from build123d import *

# Parameters (mm, degrees)
SKETCH1_W           = 127
SKETCH1_H           = 52.832
BOSS_EXTRUDE1_DEPTH = 4.7625
FILLET1_R           = 2.54
SKETCH2_R           = 2.69
CUT_EXTRUDE1_DEPTH  = 69.940093286
SKETCH3_R           = 8.250000011
CUT_EXTRUDE2_DEPTH  = 69.940093286
SKETCH4_R           = 8.255000001
SKETCH4_R_2         = 3.450513254
CUT_EXTRUDE3_DEPTH  = 69.940093286


with BuildPart() as part:
    # Sketch1 → Boss-Extrude1 (new body)
    with BuildSketch(Plane(origin=(0, 0, 0), x_dir=(1, 0, 0), z_dir=(0, 1, 0))):
        Rectangle(SKETCH1_W, SKETCH1_H)
    extrude(amount=BOSS_EXTRUDE1_DEPTH)

    # Fillet1
    fillet1_edges = [part.edges().sort_by_distance(p)[0] for p in [
        (63.5, 2.38125, 26.416),
        (-63.5, 2.38125, 26.416),
        (-63.5, 2.38125, -26.416),
        (63.5, 2.38125, -26.416),
    ]]
    fillet(fillet1_edges, radius=FILLET1_R)

    # Sketch2 → Cut-Extrude1 (cut, through all)
    with BuildSketch(Plane.XZ):
        with Locations(Location((57.15, -15.24, 0), (0, 0, 270))):
            Circle(SKETCH2_R)
        with Locations(Location((57.15, 0, 0), (0, 0, 270))):
            Circle(SKETCH2_R)
        with Locations(Location((57.15, 15.24, 0), (0, 0, 270))):
            Circle(SKETCH2_R)
    cut_extrude1 = extrude(amount=-CUT_EXTRUDE1_DEPTH, mode=Mode.SUBTRACT)

    # Mirror1: Cut-Extrude1 across plane
    add(cut_extrude1.mirror(Plane(origin=(0, 0, 0), x_dir=(0, 0, 1), z_dir=(1, 0, 0))), mode=Mode.SUBTRACT)

    # Sketch3 → Cut-Extrude2 (cut, through all)
    with BuildSketch(Plane(origin=(0, 4.7625, 0), x_dir=(1, 0, 0), z_dir=(0, 1, 0))):
        with Locations(Location((25.164289669, -5.7912, 0), (0, 0, 270))):
            Circle(SKETCH3_R)
        with Locations(Location((-0.985710355, -5.7912, 0), (0, 0, 270))):
            Circle(SKETCH3_R)
    extrude(amount=-CUT_EXTRUDE2_DEPTH, mode=Mode.SUBTRACT)

    # Sketch4 → Cut-Extrude3 (cut, through all)
    with BuildSketch(Plane(origin=(0, 4.7625, 0), x_dir=(1, 0, 0), z_dir=(0, 1, 0))):
        with Locations(Location((-26.143710331, 11.522643822, 0), (0, 0, 270))):
            Circle(SKETCH4_R)
        with Locations(Location((-26.143710331, -2.695896838, 0), (0, 0, 270))):
            Circle(SKETCH4_R_2)
    extrude(amount=-CUT_EXTRUDE3_DEPTH, mode=Mode.SUBTRACT)


solid = part.part
Part model, mm, in its own coordinate system. Round coordinates to 2 decimals unless told otherwise and drop trailing zeros. Write each loop counter-clockwise with the first axis right and the second up, starting at its lowest first coordinate (ties: lowest second). Pieces come first, ordered by that corner, then holes. Notation, with made-up numbers: M 50.25,57.5 L 105.25,57.5 A19 cw 105.25,89.5 Z; hole C -2.75,48 d8. An arc over 180 degrees is marked long. Return JSON: item names as keys, results as strings. Group by question number.
(1) Drill centre lines: probe 1 along Z at (x, y) = (-57.5, 3.1); probe 2 along X at (y, z) = (2.7, 15.24); probe 3 along X at (y, z) = (1, 1.5). Where is each one in solid material? Low to high.
(2) Pin check, flat tips, straight feed: pin 1 Ø13 at (x, z) = (25.16, 5.79) entering from -Y; pin 2 Ø4 at (x, z) = (-22, -18.5) entering from +Y. Stop position of each tip, or through.
(3) Saw through at C-C on y = 3.85. Count the separate pieces of the cut face and the enclosed holes in it, then the cut area to 3 significant figures.
(4) Two-plate mould, pull along Z, no slides. Class faces 1 (the face through (-1, 2, 26.416)), 2 (the face through (-62.78, 2.41, -25.65)), 3 (the face through (63.5, 2, 0)), 4 (the face through (-4.15, 2.41, 13.41)): +Z half, -Z half, draft (parallel to the pull), parting line (faces both ways), or undercut.
(5) Saw through at A-A on z = 15.24. Write the cut outline in (x, y), then the cut area to 3 significant figures.
(6) Saw through at B-B on x = -57.15. Write the cut outline in (y, z).
Returned:
{
 "1": {"probe 1": "-26.42 to -17.91, -12.57 to -2.67, 2.67 to 12.57, 17.91 to 26.42", "probe 2": "-63.5 to -59.84, -54.46 to 54.46, 59.84 to 63.5", "probe 3": "-63.5 to -59.38, -54.92 to -29.38, -22.91 to -8.03, 6.06 to 18.12, 32.21 to 54.92, 59.38 to 63.5"},
 "2": {"pin 1": "through", "pin 2": "y = 4.76"},
 "3": {"separate pieces": "1", "enclosed holes": "10", "area": "5,890 mm²"},
 "4": {"face 1": "+Z half", "face 2": "-Z half", "face 3": "draft", "face 4": "undercut"},
 "5": {"outline": "M -63.5,0 L -59.84,0 L -59.84,4.76 L -63.5,4.76 Z; M -54.46,0 L 54.46,0 L 54.46,4.76 L -54.46,4.76 Z; M 59.84,0 L 63.5,0 L 63.5,4.76 L 59.84,4.76 Z", "area": "554 mm²"},
 "6": {"outline": "M 0,-26.42 L 4.76,-26.42 L 4.76,-17.93 L 0,-17.93 Z; M 0,-12.55 L 4.76,-12.55 L 4.76,-2.69 L 0,-2.69 Z; M 0,2.69 L 4.76,2.69 L 4.76,12.55 L 0,12.55 Z; M 0,17.93 L 4.76,17.93 L 4.76,26.42 L 0,26.42 Z"}
}
